Input: part model. Units: mm. Frame: model coordinates. A direction names the side the tool comes from. Round coordinates to 2 decimals unless told otherwise and drop trailing zeros. Loops run counter-clockwise (first coordinate to the right, second up) from the corner with the lowest first, then second, coordinate; pieces in that order, holes last. Notation, with made-up numbers: (62.5, -9) - (107.5, -9) arc R8 ccw to (107.5, 1) - close; hole circle Ø8 at (64, 25.25). An arc over 180 degrees is marked (long way). Use CSV: the item, a comma, the result in double quotes. Start each with the question number.
1. Access query for faces 1 (the flat face through (1.28, -5.07, 2.17)), 2 (the cylindrical face through (0.9, 31.01, 2.86)), 3 (the flat face through (-10, 12, 1)), 4 (the flat face through (10, 6, -1.75)), 5 (the flat face through (-4, 16, 8)). Directions: +Z, -Z, +X, -X, +Y, -Y. A direction counts if a zero-diameter tool reaches every point of the face in a straight line with its end or side. Return the directions, or none.
2. Cut plane D-D (z = -8.25). Return loops of the section in (x, y).
3. Material intervals for probe 1 along X at (y, z) = (21, 0); probe 2 along Z at (x, y) = (1.75, 3); probe 3 along Y at (x, z) = (-6.25, -2.5), sorted ascending. Write a range as from..to.
4. Pin query (flat end, axial travel): P1, Ø2, axis at y = -3, z = 3.5, coming from the -X side; P2, Ø8, axis at y = 10, z = 4.5, coming from the -X side; P3, Ø3, axis at y = 13.5, z = -3, coming from the -X side. Return the tip coordinate at first contact, or that it passes through.
5. Cut plane C-C (x = 6.25). Return loops of the section in (y, z).
6. Cut plane A-A (y = 10.5). Return loops of the section in (x, z), and give its area (3 significant figures).
7. Pull-direction query (Z, two-part tool) for faces 6 (the flat face through (3, -10, 0)), 7 (the cylindrical face through (3.905, -5.437, -0.867)), 8 (the flat face through (1.242, -5.07, -2.193)); classes: +Z half, -Z half, draft (parallel to the pull), parting line (faces both ways), or undercut.
8. Cut plane B-B (y = 17). Return loops of the section in (x, z).
```python
from build123d import *

# Parameters (mm, degrees)
SKETCH_1_R          = 11.25
EXTRUDE_1_DEPTH     = 32
SKETCH_3_R          = 1.21
CUT_EXTRUDE_1_DEPTH = 30
SKETCH_4_R          = 4
EXTRUDE_2_DEPTH     = 10
CUT_EXTRUDE_2_DEPTH = 10
CHAMFER_1_SIZE      = 1
SKETCH_6_W          = 8
SKETCH_6_H          = 5
CUT_EXTRUDE_3_DEPTH = 45.912414765
SKETCH_7_R          = 1.6
CUT_EXTRUDE_4_DEPTH = 6
SKETCH_8_R          = 3
CUT_EXTRUDE_5_DEPTH = 2
CUT_EXTRUDE_6_DEPTH = 12


with BuildPart() as part:
    # 草图1 → 凸台-拉伸1 (new body)
    with BuildSketch(Plane(origin=(0, 0, 0), x_dir=(1, 0, 0), z_dir=(0, 1, 0))):
        with Locations(Location((0, 0, 0), (0, 0, 270))):
            Circle(SKETCH_1_R)
    extrude(amount=EXTRUDE_1_DEPTH)

    # 草图3 → 切除-拉伸1 (cut)
    with BuildSketch(Plane.XZ):
        with Locations(Location((9, 0, 0), (0, 0, 270))):
            Circle(SKETCH_3_R)
        with Locations(Location((-9, 0, 0), (0, 0, 90))):
            Circle(SKETCH_3_R)
    extrude(amount=-CUT_EXTRUDE_1_DEPTH, mode=Mode.SUBTRACT)

    # 草图4 → 凸台-拉伸2 (add)
    with BuildSketch(Plane.XZ):
        with Locations(Location((0, 0, 0), (0, 0, 90))):
            Circle(SKETCH_4_R)
    extrude(amount=EXTRUDE_2_DEPTH)

    # 草图5 → 切除-拉伸2 (cut)
    with BuildSketch(Plane.XZ.offset(10)):
        Polygon((0, -2.909845357), (2.52, -1.454922678), (2.52, 1.454922678), (0, 2.909845357), (-2.52, 1.454922678), (-2.52, -1.454922678), align=None)
    extrude(amount=-CUT_EXTRUDE_2_DEPTH, mode=Mode.SUBTRACT)

    # 倒角1
    chamfer_1_edges = [part.edges().sort_by_distance(p)[0] for p in [
        (0, 0, -4),
    ]]
    chamfer(chamfer_1_edges, length=CHAMFER_1_SIZE)

    # 草图6 → 切除-拉伸3 (cut, through all)
    with BuildSketch(Plane(origin=(0, 32, 0), x_dir=(1, 0, 0), z_dir=(0, 1, 0))):
        with Locations((0, -8.014870422)):
            Rectangle(SKETCH_6_W, SKETCH_6_H)
        with BuildLine():
            Line((4, -10.514870422), (-4, -10.514870422))
            ThreePointArc((-4, -10.514870422), (0, -11.25), (4, -10.514870422))
        make_face()
    extrude(amount=-CUT_EXTRUDE_3_DEPTH, mode=Mode.SUBTRACT)

    # 草图7 → 切除-拉伸4 (cut)
    with BuildSketch(Plane(origin=(0, 32, 0), x_dir=(1, 0, 0), z_dir=(0, 1, 0))):
        with Locations(Location((-7.361215932, 4.25, 0), (0, 0, 270))):
            Circle(SKETCH_7_R)
        with Locations(Location((7.361215932, -4.25, 0), (0, 0, 90))):
            Circle(SKETCH_7_R)
    extrude(amount=-CUT_EXTRUDE_4_DEPTH, mode=Mode.SUBTRACT)

    # 草图8 → 切除-拉伸5 (cut)
    with BuildSketch(Plane(origin=(0, 32, 0), x_dir=(1, 0, 0), z_dir=(0, 1, 0))):
        with Locations(Location((0, 0, 0), (0, 0, 270))):
            Circle(SKETCH_8_R)
    extrude(amount=-CUT_EXTRUDE_5_DEPTH, mode=Mode.SUBTRACT)

    # 草图9 → 切除-拉伸6 (cut)
    with BuildSketch(Plane.XZ):
        with BuildLine():
            ThreePointArc((-11.113055385, 1.75), (-11.25, 0), (-11.113055385, -1.75))
            Line((-11.113055385, -1.75), (-9, -1.75))
            ThreePointArc((-9, -1.75), (-10.75, 0), (-9, 1.75))
            Line((-9, 1.75), (-11.113055385, 1.75))
        make_face()
        with BuildLine():
            ThreePointArc((-9, 1.75), (-10.75, 0), (-9, -1.75))
            Line((-9, -1.75), (-9, -1.21))
            ThreePointArc((-9, -1.21), (-10.21, 0), (-9, 1.21))
            Line((-9, 1.21), (-9, 1.75))
        make_face()
        with BuildLine():
            Line((-9, -1.21), (-9, -1.75))
            ThreePointArc((-9, -1.75), (-7.762563133, -1.237436867), (-7.25, 0))
            ThreePointArc((-7.25, 0), (-7.762563133, 1.237436867), (-9, 1.75))
            Line((-9, 1.75), (-9, 1.21))
            ThreePointArc((-9, 1.21), (-8.144400795, 0.855599205), (-7.79, 0))
            ThreePointArc((-7.79, 0), (-8.144400795, -0.855599205), (-9, -1.21))
        make_face()
        with BuildLine():
            ThreePointArc((9, 1.75), (7.25, 0), (9, -1.75))
            Line((9, -1.75), (9, -1.21))
            ThreePointArc((9, -1.21), (7.79, 0), (9, 1.21))
            Line((9, 1.21), (9, 1.75))
        make_face()
        with BuildLine():
            Line((9, -1.21), (9, -1.75))
            ThreePointArc((9, -1.75), (10.237436867, -1.237436867), (10.75, 0))
            ThreePointArc((10.75, 0), (10.237436867, 1.237436867), (9, 1.75))
            Line((9, 1.75), (9, 1.21))
            ThreePointArc((9, 1.21), (9.855599205, 0.855599205), (10.21, 0))
            ThreePointArc((10.21, 0), (9.855599205, -0.855599205), (9, -1.21))
        make_face()
        with BuildLine():
            Line((9, -1.75), (11.113055385, -1.75))
            ThreePointArc((11.113055385, -1.75), (11.25, 0), (11.113055385, 1.75))
            Line((11.113055385, 1.75), (9, 1.75))
            ThreePointArc((9, 1.75), (10.237436867, 1.237436867), (10.75, 0))
            ThreePointArc((10.75, 0), (10.237436867, -1.237436867), (9, -1.75))
        make_face()
    extrude(amount=-CUT_EXTRUDE_6_DEPTH, mode=Mode.SUBTRACT)


solid = part.part
```
Established:
1,face 1,"-Y"
1,face 2,"+Y"
1,face 3,"-X, -Y"
1,face 4,"+X, -Y"
1,face 5,"+Z, +Y, -Y"
2,outline,"(-7.65, 0) - (7.65, 0) - (7.65, 32) - (-7.65, 32) - close"
3,probe 1,"x = -11.25..-10.21, -7.79..7.79, 10.21..11.25"
3,probe 2,"z = -11.11..5.51"
3,probe 3,"y = 0..32"
4,P1,"stops at x = -3.12"
4,P2,"stops at x = -11.2"
4,P3,"stops at x = -11.15"
5,outline,"(0, -9.35) - (32, -9.35) - (32, 3.1) - (26, 3.1) - (26, 5.4) - (32, 5.4) - (32, 9.35) - (0, 9.35) - close"
6,outline,"(-11.11, -1.75) arc R11.25 ccw to (11.11, -1.75) - (9, -1.75) arc R1.75 cw to (9, 1.75) - (11.11, 1.75) arc R11.25 ccw to (4, 10.51) - (4, 5.51) - (-4, 5.51) - (-4, 10.51) arc R11.25 ccw to (-11.11, 1.75) - (-9, 1.75) arc R1.75 cw to (-9, -1.75) - close"
6,area,"329 mm2"
7,face 6,"draft"
7,face 7,"parting line"
7,face 8,"undercut"
8,outline,"(-4, 5.51) - (-4, 10.51) arc R11.25 ccw (long way) to (4, 10.51) - (4, 5.51) - close; hole circle Ø2.42 at (-9, 0); hole circle Ø2.42 at (9, 0)"
